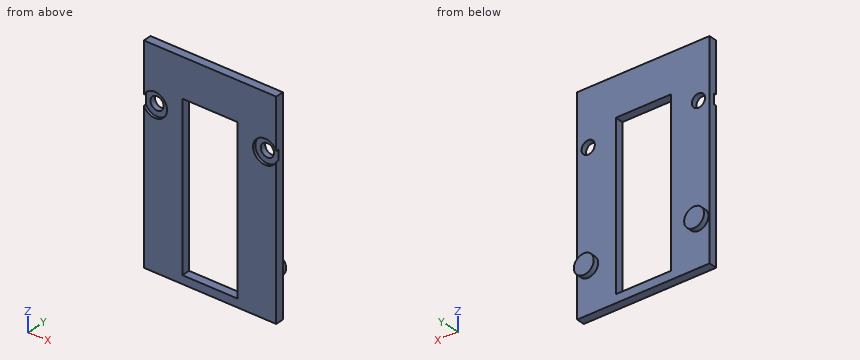
from build123d import *

# Parameters (mm, degrees)
ESQUISSE1_W           = 24
ESQUISSE1_H           = 38
ESQUISSE1_W_2         = 10
ESQUISSE1_H_2         = 29.5
SHAPE_DEPTH           = 1.5
ESQUISSE2_R           = 1.2
VISHOLES_DEPTH        = 1.5
ESQUISSE3_R           = 1.8
LOCKERS_DEPTH         = 1
ESQUISSE4_R           = 2.2
SCREWHATREMOVER_DEPTH = 0.5


with BuildPart() as part:
    # Esquisse1 → Shape (new body)
    with BuildSketch(Plane(origin=(0, 0, 0), x_dir=(1, 0, 0), z_dir=(0, 1, 0))):
        Rectangle(ESQUISSE1_W, ESQUISSE1_H)
        with Locations((0, 2.75)):
            Rectangle(ESQUISSE1_W_2, ESQUISSE1_H_2, mode=Mode.SUBTRACT)
    extrude(amount=SHAPE_DEPTH)

    # Esquisse2 → VisHoles (cut)
    with BuildSketch(Plane(origin=(0, 1.5, 0), x_dir=(1, 0, 0), z_dir=(0, 1, 0))):
        with Locations(Location((10, -9, 0), (0, 0, 270))):
            Circle(ESQUISSE2_R)
    visholes = extrude(amount=-VISHOLES_DEPTH, mode=Mode.SUBTRACT)

    # Esquisse3 → Lockers (add)
    with BuildSketch(Plane(origin=(0, 1.5, 0), x_dir=(1, 0, 0), z_dir=(0, 1, 0))):
        with Locations(Location((10, 11, 0), (0, 0, 90))):
            Circle(ESQUISSE3_R)
    lockers = extrude(amount=LOCKERS_DEPTH)

    # Esquisse4 → ScrewHatRemover (cut)
    with BuildSketch(Plane(origin=(0, 0, 0), x_dir=(1, 0, 0), z_dir=(0, 1, 0))):
        with Locations((10, -9)):
            Circle(ESQUISSE4_R)
    screwhatremover = extrude(amount=SCREWHATREMOVER_DEPTH, mode=Mode.SUBTRACT)

    # Symétrie1: VisHoles, Lockers, ScrewHatRemover across plane
    add(visholes.mirror(Plane(origin=(0, 0, 0), x_dir=(0, 0, 1), z_dir=(1, 0, 0))), mode=Mode.SUBTRACT)
    add(lockers.mirror(Plane(origin=(0, 0, 0), x_dir=(0, 0, 1), z_dir=(1, 0, 0))))
    add(screwhatremover.mirror(Plane(origin=(0, 0, 0), x_dir=(0, 0, 1), z_dir=(1, 0, 0))), mode=Mode.SUBTRACT)


solid = part.part
Read the model definition and answer for the solid it produces. Units are mm, in the model's axes. Round coordinates to 2 decimals unless told otherwise and drop trailing zeros. Write each loop counter-clockwise with the first axis right and the second up, starting at its lowest first coordinate (ties: lowest second). Pieces come first, ordered by that corner, then holes.
Q1. Flat-ended cylindrical pins translate along their axes: P1, Ø7, axis at x = -4.5, z = -3, coming from the +Y side; P2, Ø2, axis at x = -10.5, z = 9.5, coming from the -Y side; P3, Ø4.5, axis at x = 11, z = 9.5, coming from the -Y side. Find the tip coordinate at first contact, or state that the pin passes through.
Values:
P1: stops at y = 1.5
P2: stops at y = 0.5
P3: stops at y = 0
Q2. Find section D-D on x = 4.5. Determine the outline of the cut face in (y, z).
Values:
outline: (0, -19) - (1.5, -19) - (1.5, -17.5) - (0, -17.5) - close; (0, 12) - (1.5, 12) - (1.5, 19) - (0, 19) - close
Q3. Find section C-C on z = 9. Determine the outline of the cut face in (x, y).
Values:
outline: (-12, 0.5) - (-11.2, 0.5) - (-11.2, 1.5) - (-12, 1.5) - close; (-8.8, 0.5) - (-7.8, 0.5) - (-7.8, 0) - (-5, 0) - (-5, 1.5) - (-8.8, 1.5) - close; (5, 0) - (7.8, 0) - (7.8, 0.5) - (8.8, 0.5) - (8.8, 1.5) - (5, 1.5) - close; (11.2, 0.5) - (12, 0.5) - (12, 1.5) - (11.2, 1.5) - close
Q4. Find section A-A on z = -13.5. Determine the outline of the cut face in (x, y).
Values:
outline: (-12, 0) - (-5, 0) - (-5, 1.5) - (-12, 1.5) - close; (5, 0) - (12, 0) - (12, 1.5) - (5, 1.5) - close
Q5. Straight lines are drawn through the part: line 1 (Z direction, x = -3, y = 0.55); line 2 (X direction, y = 0.55, z = 2); line 3 (Z direction, x = -10, y = 1.15). For each, find the intervals that lie inside material, in ascending order.
Values:
line 1: z = -19 to -17.5, 12 to 19
line 2: x = -12 to -5, 5 to 12
line 3: z = -19 to 7.8, 10.2 to 19
Q6. Find section B-B on y = 0.95. Determine the outline of the cut face in (x, z), and give its area (3 significant figures).
Values:
outline: (-12, -19) - (12, -19) - (12, 19) - (-12, 19) - close; hole circle Ø2.4 at (-10, 9); hole (-5, -17.5) - (5, -17.5) - (5, 12) - (-5, 12) - close; hole circle Ø2.4 at (10, 9)
area: 608 mm2
